The drawing under review shows one solid part. Ordinate dimensions are in mm from its lowest x, y, z. Round coordinates to 2 decimals unless told otherwise and drop trailing zeros. Order: outer loops, then holes, each group sorted by start corner. A loop starts at its lowest first (then second) coordinate and runs counter-clockwise, first axis right, second up. Notation, with made-up numbers: M -6.5,-14.5 L 0.5,-14.5 A30 cw 0.5,23.5 Z; hole C 43.25,-30.5 d8. An arc over 180 degrees is marked long. Write item = value, one per line. Start each with the question number.
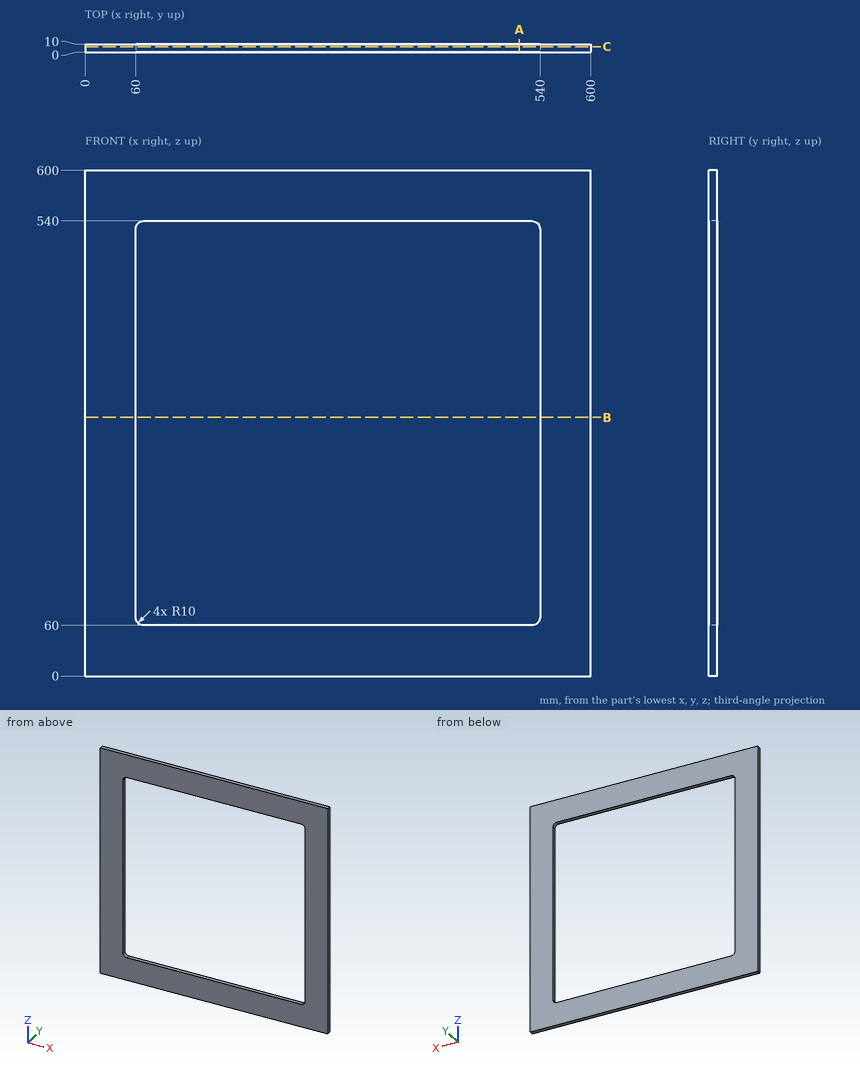
(1) Consider section B-B, the plane z = 307. Write out the cut boundary in (x, y), then the cut area to 3 significant figures.
(2) Consider section C-C, the plane y = 7. Write out the cut boundary in (x, z).
(3) Consider section A-A, the plane x = 515.5. Write out the cut boundary in (y, z), then the cut area to 3 significant figures.
(4) For line 1 along Z through (x, y) = (372, 0.75), list the stretches that pass through material, from the lowest coordinate up. Write a range as [from, to].
Completed:
q1.outline = M 0,0 L 60,0 L 60,10 L 0,10 Z; M 540,0 L 600,0 L 600,10 L 540,10 Z
q1.area = 1,200 mm2
q2.outline = M 0,0 L 600,0 L 600,600 L 0,600 Z; hole M 60,70 A10 ccw 70,60 L 530,60 A10 ccw 540,70 L 540,530 A10 ccw 530,540 L 70,540 A10 ccw 60,530 Z
q3.outline = M 0,0 L 10,0 L 10,60 L 0,60 Z; M 0,540 L 10,540 L 10,600 L 0,600 Z
q3.area = 1,200 mm2
q4.line_1 = [0, 60], [540, 600]
